Build history of the part. All positions in model axes, mm. Coordinates: 2 decimals unless noted, no trailing zeros. Write each loop counter-clockwise with the first axis right and the second up, starting at its lowest first coordinate (ties: lowest second). Pieces come first, ordered by that corner, then holes.
Autodesk Inventor part; units mm, degrees
ref_plane "YZ Plane" through (0, 0, 0) normal (1, 0, 0) x (0, 1, 0)
ref_plane "XZ Plane" through (0, 0, 0) normal (0, 1, 0) x (-1, 0, 0)
ref_plane "XY Plane" through (0, 0, 0) normal (0, 0, 1) x (1, 0, 0)
sketch "Sketch1" plane through (0, 0, 0) normal (0, 1, 0) x (-1, 0, 0)
  circle A0 centre (0, 0) radius 273.05
  circle A1 centre (0, 0) radius 242.8875
  dimension "d0" = 546.1
  dimension "d1" = 485.775
extrude "Extrusion1" add sketch "Sketch1" along normal blind 25.4
sketch "Sketch2" plane through (0, 25.4, 0) normal (0, 1, 0) x (1, 0, 0)
  circle A0 centre (0, 0) radius 247.65
  circle A1 centre (0, 0) radius 252.4125
  dimension "d4" = 495.3
  dimension "d5" = 504.825
extrude "Extrusion2" cut sketch "Sketch2" against normal blind 3.175
sketch "Sketch3" plane through (0, 25.4, 0) normal (0, 1, 0) x (1, 0, 0)
  line L0 (0, 0) -> (-265.25, 0) construction
  dimension "d8" = 265.25
hole "Hole1" at (-265.25, 25.4, 0) direction (0, -1, 0) diameter 6.1976 end up to surface
pattern_circular "Circular Pattern1" count 12 over 360 about axis through (0, -10, 0) along (0, 1, 0) of "Hole1"
sketch "Sketch4" plane through (0, 0, 0) normal (0, -1, 0) x (1, 0, 0)
  circle A0 centre (0, 0) radius 242.8875
  circle A1 centre (0, 0) radius 246.0625
  dimension "d19" = 485.775
  dimension "d20" = 492.125
extrude "Extrusion3" add sketch "Sketch4" along normal blind 431.8
sketch "Sketch5" plane through (0, -431.8, 0) normal (0, -1, 0) x (1, 0, 0)
  circle A0 centre (0, 0) radius 273.05
  circle A1 centre (0, 0) radius 242.8875
  dimension "d24" = 546.1
  dimension "d23" = 485.775
extrude "Extrusion4" add sketch "Sketch5" along normal blind 25.4
sketch "Sketch7" plane through (0, -457.2, 0) normal (0, -1, 0) x (-1, 0, 0)
  line L0 (0, 0) -> (-265.25, 0) construction
  dimension "d34" = 265.25
hole "Hole2" at (265.25, -457.2, 0) direction (0, 1, 0) diameter 8.9916 end up to surface
pattern_circular "Circular Pattern2" count 12 over 360 about axis through (0, 0, 0) along (0, -1, 0) of "Hole2"
properties part number "vacuum jacket"
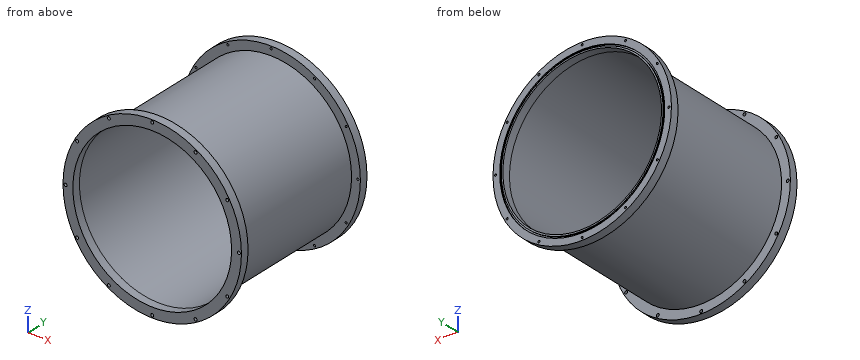
(1) Slice it at A-A, the plane x = -209.5. List the corners of the cut face in (y, z) (3 decimals), and give its area (3 significant figures).
(2) Slice it at C-C, the plane y = -104. List the corners of the cut face in (x, z) (1 decimal), and give its area (3 significant figures).
(3) Probe L1, parallel to Z at x = 0, y = 24.35; L2, parallel to Y at x = 168.5, z = -192; L3, parallel to Z at x = 115, y = -21.5. List the from-to ranges inside material, lowest first.
(4) Flat gauge pins, fed straight in: P1, Ø5.5, axis at x = -132.62, z = -229.71, coming from the +Y side; P2, Ø2, axis at y = -401, z = 41, coming from the +X side; P3, Ø7, axis at x = -229.71, z = 132.62, coming from the -Y side; P4, Ø4, axis at x = -182, y = -201, coming from the +Z side. Where does each tip first touch, or does it go through?
Results:
1. outline: (-457.2, -175.117) - (-431.8, -175.117) - (-431.8, -129.06) - (0, -129.06) - (0, -175.117) - (25.4, -175.117) - (25.4, -140.79) - (22.225, -140.79) - (22.225, -132.062) - (25.4, -132.062) - (25.4, -122.899) - (-457.2, -122.899) - close; (-457.2, 122.899) - (25.4, 122.899) - (25.4, 132.062) - (22.225, 132.062) - (22.225, 140.79) - (25.4, 140.79) - (25.4, 175.117) - (0, 175.117) - (0, 129.06) - (-431.8, 129.06) - (-431.8, 175.117) - (-457.2, 175.117) - close
1. area: 10,600 mm2
2. outline: circle Ø492.1 at (0, 0); hole circle Ø485.8 at (0, 0)
2. area: 4,880 mm2
3. L1: z = -273.05 to -268.35, -262.15 to -252.41, -247.65 to -242.89, 242.89 to 247.65, 252.41 to 262.15, 268.35 to 273.05
3. L2: y = -457.2 to -431.8, 0 to 25.4
3. L3: z = -217.54 to -213.94, 213.94 to 217.54
4. P1: passes through
4. P2: stops at x = 242.79
4. P3: stops at y = 0
4. P4: stops at z = 167.77
